Geometry check sheet. Reference: the model listing, model coordinates, mm. Round coordinates to 2 decimals unless told otherwise and drop trailing zeros. Write each loop counter-clockwise with the first axis right and the second up, starting at its lowest first coordinate (ties: lowest second). Pieces come first, ordered by that corner, then holes.
Autodesk Inventor part; units mm, degrees
ref_plane "YZ Plane" through (0, 0, 0) normal (1, 0, 0) x (0, 1, 0)
ref_plane "XZ Plane" through (0, 0, 0) normal (0, 1, 0) x (-1, 0, 0)
ref_plane "XY Plane" through (0, 0, 0) normal (0, 0, 1) x (1, 0, 0)
sketch "Sketch1" plane through (0, 0, 0) normal (0, 0, 1) x (1, 0, 0)
  line L0 (-15.6633, 0) -> (44.0267, 0)
  line L1 (44.0267, 0) -> (44.0267, 16.51)
  line L2 (44.0267, 16.51) -> (-15.6633, 16.51)
  line L3 (-15.6633, 16.51) -> (-15.6633, 0)
  point P0 (0, 0)
  dimension "d0" = 16.51
  dimension "d1" = 59.69
extrude "Extrusion1" add sketch "Sketch1" along normal mid plane 101.6
sketch "Sketch2" plane through (-9.3133, 16.51, 50.8) normal (0, 1, 0) x (1, 0, 0)
  line L0 (-6.35, 101.6) -> (-6.35, 0)
  line L1 (53.34, 0) -> (-6.35, 0)
  line L2 (53.34, 101.6) -> (53.34, 0)
  line L3 (-6.35, 101.6) -> (53.34, 101.6)
  line L4 (-6.35, 0) -> (-6.35, 101.6343) construction
  line L5 (-6.35, 101.6343) -> (53.34, 101.6343) construction
  line L6 (53.34, 101.6343) -> (53.34, 0) construction
  line L7 (53.34, 0) -> (-6.35, 0) construction
sketch "Sketch3" plane through (-15.6633, 0, 50.8) normal (0, -1, 0) x (1, 0, 0)
  line L0 (59.69, -101.6) -> (59.69, 0)
  line L1 (0, 0) -> (59.69, 0)
  line L2 (0, 0) -> (0, -101.6)
  line L3 (59.69, -101.6) -> (0, -101.6)
  line L4 (0, 0) -> (59.69, 0)
  line L5 (59.69, 0) -> (59.6518, -101.6224) construction
  line L6 (59.6518, -101.6224) -> (0, -101.6) construction
  line L7 (0, -101.6) -> (0.0382, 0.0224) construction
  line L8 (0.0382, 0.0224) -> (59.69, 0) construction
  point P0 (15.6633, -50.8)
sketch "Sketch4" plane through (44.0267, 0, 50.8) normal (0, 0, 1) x (1, 0, 0)
  line L0 (-59.69, 0) -> (0, 0)
  line L1 (0, 0) -> (0, 16.51)
  line L2 (0, 16.51) -> (-59.69, 16.51)
  line L3 (-59.69, 16.51) -> (-59.69, 0)
  line L4 (0, 16.51) -> (-59.69, 16.51)
  line L5 (-59.69, 16.51) -> (0.0244, 16.4214) construction
  line L6 (0.0244, 16.4214) -> (0, 0) construction
  line L7 (0, 0) -> (-59.7144, 0.0886) construction
  line L8 (-59.7144, 0.0886) -> (-59.69, 16.51) construction
sketch "Sketch5" plane through (0, 0, -50.8) normal (0, 0, -1) x (-1, 0, 0)
  line L0 (-44.0267, 0) -> (15.6633, 0)
  line L1 (15.6633, 0) -> (15.6633, 16.51)
  line L2 (15.6633, 16.51) -> (-44.0267, 16.51)
  line L3 (-44.0267, 16.51) -> (-44.0267, 0)
  line L4 (-44.0267, 16.51) -> (15.6633, 16.51)
  line L5 (-44.0267, 16.51) -> (15.6877, 16.4214) construction
  line L6 (15.6877, 16.4214) -> (15.6633, 0) construction
  line L7 (15.6633, 0) -> (-44.051, 0.0886) construction
  line L8 (-44.051, 0.0886) -> (-44.0267, 16.51) construction
  point P0 (0, 0)
sketch "Sketch6" plane through (44.0267, 0, 50.8) normal (1, 0, 0) x (0, 0, -1)
  line L0 (101.6, 16.51) -> (0, 16.51)
  line L1 (0, 0) -> (0, 16.51)
  line L2 (101.6, 0) -> (0, 0)
  line L3 (101.6, 16.51) -> (101.6, 0)
  line L4 (101.6, 16.51) -> (0, 16.51)
  line L5 (0, 16.51) -> (101.6, 16.51) construction
  line L6 (101.6, 16.51) -> (101.6, 0) construction
  line L7 (101.6, 0) -> (0, 0) construction
  line L8 (0, 0) -> (0, 16.51) construction
  point P0 (50.8, 0)
  dimension "d174" = 101.6
  dimension "d175" = 16.51
sketch "Sketch7" plane through (-15.6633, 0, 50.8) normal (-1, 0, 0) x (0, 0, 1)
  line L0 (-101.6, 16.51) -> (-101.6, 0)
  line L1 (-101.6, 16.51) -> (0, 16.51) construction
  line L2 (0, 16.51) -> (0, 0) construction
  line L3 (0, 0) -> (-101.6, 0) construction
  line L4 (-101.6, 0) -> (-101.6, 16.51) construction
  point P0 (-50.8, 0)
fillet "Fillet2" radius 7.62 4 edges at (44.0267, 16.51, 0) (44.0267, 0, 0) (-15.6633, 16.51, 0) (-15.6633, 0, 0)
decal "Decal1"
decal "Decal2"
decal "Decal3"
decal "Decal4"
decal "Decal5"
decal "Decal6"
properties part number "Tenergy NiMH Battery Pack 9.6V 2000mAh High Capacity Rechargeable RC Battery"
1. Scan lines: line 1 along Y through (x, z) = (-8.5, -38); line 2 along X through (y, z) = (9.25, 25.5); line 3 along X through (y, z) = (14, -45). Record each from-to range of solid material in increasing order.
2. Section check B-B (y = 14). Record the cut outline in (x, z), plus the area to 3 significant figures.
3. Section check A-A (z = 36). Record the cut outline in (x, y), plus the area to 3 significant figures.
4. Section check C-C (y = 4.5). Record the cut outline in (x, z).
Results below:
1. line 1: y = 0.01 to 16.5
1. line 2: x = -15.65 to 44.02
1. line 3: x = -13.7 to 42.06
2. outline: (-13.7, -50.8) - (42.06, -50.8) - (42.06, 50.8) - (-13.7, 50.8) - close
2. area: 5,660 mm2
3. outline: (-15.66, 7.62) arc R7.62 ccw to (-8.04, 0) - (36.41, 0) arc R7.62 ccw to (44.03, 7.62) - (44.03, 8.89) arc R7.62 ccw to (36.41, 16.51) - (-8.04, 16.51) arc R7.62 ccw to (-15.66, 8.89) - close
3. area: 936 mm2
4. outline: (-15, -50.8) - (43.36, -50.8) - (43.36, 50.8) - (-15, 50.8) - close
